For this review, take the finished solid that the model builds, in its own axes (mm). A direction names the side the tool comes from. Give positions to 0.01 mm unless a question says otherwise; leave off trailing zeros. Loops run counter-clockwise (first coordinate to the right, second up) from the corner with the lowest first, then second, coordinate; pieces in that order, holes last. Notation, with made-up numbers: (4.5, -13.75) - (9.5, -13.75) arc R31 ccw to (9.5, 18.25) - close; hole circle Ø11 at (-37.5, 6). An arc over 180 degrees is marked (long way). Put each result on its own line as item: value.
from build123d import *

# Parameters (mm, degrees)
SKETCH1_W           = 44.958
SKETCH1_H           = 44.958
SKETCH1_W_2         = 38.608
SKETCH1_H_2         = 38.608
BOSS_EXTRUDE1_DEPTH = 11.43
CHAMFER1_SIZE       = 0.508
CHAMFER1_SIZE2      = 5.80646657


with BuildPart() as part:
    # Sketch1 → Boss-Extrude1 (new body)
    with BuildSketch(Plane(origin=(0, 0, 0), x_dir=(1, 0, 0), z_dir=(0, 1, 0))):
        Rectangle(SKETCH1_W, SKETCH1_H)
        Rectangle(SKETCH1_W_2, SKETCH1_H_2, mode=Mode.SUBTRACT)
    extrude(amount=BOSS_EXTRUDE1_DEPTH)

    # Chamfer1
    chamfer1_edges = [part.edges().sort_by_distance(p)[0] for p in [
        (19.304, 11.43, 0),
        (0, 11.43, -19.304),
        (-19.304, 11.43, 0),
        (0, 11.43, 19.304),
    ]]
    chamfer1_side = [part.faces().sort_by_distance(p)[0] for p in [
        (0, 11.43, 21.843197867),
    ]]
    chamfer(chamfer1_edges, length=CHAMFER1_SIZE, length2=CHAMFER1_SIZE2, reference=chamfer1_side[0])


solid = part.part
1) Draft analysis for pull direction Y (two halves, no side actions). For faces 4 (the face through (0, 6, 22.479)), 5 (the face through (-20, 0, 0)), 6 (the face through (-19.554, 8.486, 0.277)), state which applies: pulls with the +Y half, pulls with the -Y half, needs draft (parallel to the pull), parting line crosses it, or undercut.
Geometry check:
face 4: needs draft
face 5: pulls with the -Y half
face 6: pulls with the +Y half
2) Take a section at C-C on y = 2.5. State the section outline as (x, z) points.
Geometry check:
outline: (-22.48, -22.48) - (22.48, -22.48) - (22.48, 22.48) - (-22.48, 22.48) - close; hole (-19.3, -19.3) - (19.3, -19.3) - (19.3, 19.3) - (-19.3, 19.3) - close
3) Take a section at A-A on z = -18.5. State the section outline as (x, y) points.
Geometry check:
outline: (-22.48, 0) - (-19.3, 0) - (-19.3, 5.62) - (-19.81, 11.43) - (-22.48, 11.43) - close; (19.3, 0) - (22.48, 0) - (22.48, 11.43) - (19.81, 11.43) - (19.3, 5.62) - close
4) Wall thickness on line 1 (X direction, y = 5.25, z = 15.5); line 2 (X direction, y = 7, z = 7): over which ranges is each line inside the solid? List them lowest first.
Geometry check:
line 1: x = -22.48 to -19.3, 19.3 to 22.48
line 2: x = -22.48 to -19.42, 19.42 to 22.48
5) For faces 1 (the face through (22.479, 6, 0)), 2 (the face through (-0.277, 8.486, 19.554)), 3 (the face through (-19.304, 3, 0)), list the 3-axis set-ups (+Z, -Z, +X, -X, +Y, -Y) from which the entire face can be reached by the end or side of a thin tool; tool diameter is ignored.
Geometry check:
face 1: +Z, -Z, +X, +Y, -Y
face 2: +Y
face 3: +Y, -Y
6) Take a section at D-D on y = 7. State the section outline as (x, z) points.
Geometry check:
outline: (-22.48, -22.48) - (22.48, -22.48) - (22.48, 22.48) - (-22.48, 22.48) - close; hole (-19.42, -19.42) - (19.42, -19.42) - (19.42, 19.42) - (-19.42, 19.42) - close
7) Take a section at B-B on x = 4.5. State the section outline as (y, z) points.
Geometry check:
outline: (0, -22.48) - (11.43, -22.48) - (11.43, -19.81) - (5.62, -19.3) - (0, -19.3) - close; (0, 19.3) - (5.62, 19.3) - (11.43, 19.81) - (11.43, 22.48) - (0, 22.48) - close
